from build123d import *

# Parameters (mm, degrees)
SKETCH1_W               = 31.224798093
SKETCH1_H               = 19.847341298
BOSS_EXTRUDE1_DEPTH     = 3.302
SKETCH2_R               = 1.2065
CUT_EXTRUDE1_DEPTH      = 19.847341298
SKETCH3_W               = 6.232143457
SKETCH3_H               = 2.69875
CUT_EXTRUDE2_DEPTH      = 19.847341298
CUT_EXTRUDE4_DEPTH      = 19.847341298
SKETCH6_W               = 7.202949523
SKETCH6_H               = 3.302
CUT_EXTRUDE5_DEPTH      = 19.847341298
SKETCH7_R               = 1.27
CUT_EXTRUDE6_DEPTH      = 0.60325
MIRROR4_COPY_1_SKETCH_R = 1.27
MIRROR4_COPY_1_DEPTH    = 0.60325


with BuildPart() as part:
    # Sketch1 → Boss-Extrude1 (new body)
    with BuildSketch(Plane.XY):
        with Locations((-25.734325238, 15.946701424)):
            Rectangle(SKETCH1_W, SKETCH1_H)
    extrude(amount=BOSS_EXTRUDE1_DEPTH)

    # Sketch2 → Cut-Extrude1 (cut)
    with BuildSketch(Plane.XZ.offset(-6.023030775)):
        with Locations((-25.734325238, 0)):
            Circle(SKETCH2_R)
    extrude(amount=-CUT_EXTRUDE1_DEPTH, mode=Mode.SUBTRACT)

    # Sketch3 → Cut-Extrude2 (cut)
    with BuildSketch(Plane.XZ.offset(-6.023030775)):
        with Locations((-31.390396967, 1.952625)):
            Rectangle(SKETCH3_W, SKETCH3_H)
    cut_extrude2 = extrude(amount=-CUT_EXTRUDE2_DEPTH, mode=Mode.SUBTRACT)

    # Mirror1: Cut-Extrude2 across plane
    add(cut_extrude2.mirror(Plane.ZY.offset(25.734325238)), mode=Mode.SUBTRACT)

    # Sketch5 → Cut-Extrude4 (cut)
    with BuildSketch(Plane.XZ.offset(-6.023030775)):
        with BuildLine():
            Line((-28.274325238, 0.60325), (-28.274325238, 3.302))
            Line((-28.274325238, 3.302), (-23.194325238, 3.302))
            Line((-23.194325238, 3.302), (-23.194325238, 0.60325))
            ThreePointArc((-23.194325238, 0.60325), (-25.734325238, 3.14325), (-28.274325238, 0.60325))
        make_face()
    extrude(amount=-CUT_EXTRUDE4_DEPTH, mode=Mode.SUBTRACT)

    # Sketch6 → Cut-Extrude5 (cut)
    with BuildSketch(Plane.XZ.offset(-6.023030775)):
        with Locations((-37.745249523, 1.651)):
            Rectangle(SKETCH6_W, SKETCH6_H)
    cut_extrude5 = extrude(amount=-CUT_EXTRUDE5_DEPTH, mode=Mode.SUBTRACT)

    # Mirror2: Cut-Extrude5 across plane
    add(cut_extrude5.mirror(Plane.ZY.offset(25.734325238)), mode=Mode.SUBTRACT)

    # Sketch7 → Cut-Extrude6 (cut)
    with BuildSketch(Plane.XY.offset(0.60325)):
        with Locations((-30.814325238, 11.103030775)):
            Circle(SKETCH7_R)
    cut_extrude6 = extrude(amount=-CUT_EXTRUDE6_DEPTH, mode=Mode.SUBTRACT)

    # Mirror3: Cut-Extrude6 across plane
    add(cut_extrude6.mirror(Plane(origin=(0, 15.946701424, 0), x_dir=(0, 0, 1), z_dir=(0, -1, 0))), mode=Mode.SUBTRACT)

    # Mirror4: Cut-Extrude6 across plane
    add(cut_extrude6.mirror(Plane.ZY.offset(25.734325238)), mode=Mode.SUBTRACT)

    # Mirror4 copy 1 sketch → Mirror4 copy 1 (cut)
    with BuildSketch(Plane(origin=(-51.468650475, 31.893402848, 0.60325), x_dir=(-1, 0, 0), z_dir=(0, 0, 1))):
        with Locations((-30.814325238, 11.103030775)):
            Circle(MIRROR4_COPY_1_SKETCH_R)
    extrude(amount=-MIRROR4_COPY_1_DEPTH, mode=Mode.SUBTRACT)


solid = part.part
Design review of the part built by this model. Coordinates are the model's own, in mm. A direction names the side the tool comes from. Round coordinates to 2 decimals unless told otherwise and drop trailing zeros. Write each loop counter-clockwise with the first axis right and the second up, starting at its lowest first coordinate (ties: lowest second). Pieces come first, ordered by that corner, then holes. Notation, with made-up numbers: (-13, 0.5) - (33, 0.5) arc R17 cw to (33, 21.5) - close; hole circle Ø2 at (10.5, -15). An arc over 180 degrees is marked (long way). Use a Markdown table: item, result. Add a question column.
1. Mouldability with a two-part tool opening along Y and no side actions: class faces 1 (the face through (-26, 6.023, 2)), 2 (the face through (-31, 16, 0)), 3 (the face through (-31.09, 9.863, 0.306)) as +Y half, -Y half, draft (parallel to the pull), parting line (faces both ways), or undercut.
2. Clearance check with flat-ended pins moving along their axes: pin 1 (4 mm diameter, centred on x = -20.65, y = 20.79, fed in from +Z); pin 2 (1 mm diameter, centred on y = 17, z = 1.5, fed in from -X); pin 3 (1.5 mm diameter, centred on x = -25.5, y = 16.5, fed in from -Z). State where each tip first meets the part, or that it passes through.
3. We need section B-B (y = 24). State the section outline as (x, z) points, then the cut area to 3 significant figures.
4. For faces 4 (the face through (-31, 16, 0.603)), 5 (the face through (-20.49, 19.53, 0.31)), 6 (the face through (-20, 16, 0.603)), list the 3-axis set-ups (+Z, -Z, +X, -X, +Y, -Y) from which the entire face can be reached by the end or side of a thin tool; tool diameter is ignored.
5. We need section C-C (x = -21). State the section outline as (y, z) points, then the cut area to 3 significant figures.
6. We need section A-A (z = 0.3). State the section outline as (x, y) points, then the cut area to 3 significant figures.
7. Wall thickness on probe 1 along Y at (x, z) = (-19.5, 0.35); probe 2 along Y at (x, z) = (-30.75, 0.3); probe 3 along Z at (x, y) = (-32.25, 21.5): over which ranges is each line inside the solid? List them lowest first.
8. We need section D-D (y = 21.5). State the section outline as (x, z) points, then the cut area to 3 significant figures.
Output:
| question | item | result |
|---|---|---|
| 1 | face 1 | -Y half |
| 1 | face 2 | draft |
| 1 | face 3 | undercut |
| 2 | pin 1 | stops at z = 0.6 |
| 2 | pin 2 | stops at x = -28.24 |
| 2 | pin 3 | stops at z = 0.7 |
| 3 | outline | (-34.14, 0) - (-26.94, 0) arc R1.21 cw to (-24.53, 0) - (-17.32, 0) - (-17.32, 0.6) - (-23.19, 0.6) arc R2.54 ccw to (-28.27, 0.6) - (-34.14, 0.6) - close |
| 3 | area | 18.0 mm2 |
| 4 | face 4 | +Z, -X, +Y, -Y |
| 4 | face 5 | +Z, -Z |
| 4 | face 6 | +Z, +X, +Y, -Y |
| 5 | outline | (6.02, 0) - (9.88, 0) - (9.88, 0.6) - (6.02, 0.6) - close; (12.33, 0) - (19.57, 0) - (19.57, 0.6) - (12.33, 0.6) - close; (22.01, 0) - (25.87, 0) - (25.87, 0.6) - (22.01, 0.6) - close |
| 5 | area | 9.02 mm2 |
| 6 | outline | (-34.14, 6.02) - (-26.9, 6.02) - (-26.9, 25.87) - (-34.14, 25.87) - close; (-24.57, 6.02) - (-17.32, 6.02) - (-17.32, 25.87) - (-24.57, 25.87) - close; hole circle Ø2.54 at (-30.81, 11.1); hole circle Ø2.54 at (-30.81, 20.79); hole circle Ø2.54 at (-20.65, 11.1); hole circle Ø2.54 at (-20.65, 20.79) |
| 6 | area | 267 mm2 |
| 7 | probe 1 | y = 6.02 to 10.57, 11.63 to 20.26, 21.32 to 25.87 |
| 7 | probe 2 | y = 6.02 to 9.83, 12.37 to 19.52, 22.06 to 25.87 |
| 7 | probe 3 | z = 0 to 0.6 |
| 8 | outline | (-34.14, 0) - (-31.87, 0) - (-31.87, 0.6) - (-34.14, 0.6) - close; (-29.76, 0) - (-26.94, 0) arc R1.21 cw to (-24.53, 0) - (-21.71, 0) - (-21.71, 0.6) - (-23.19, 0.6) arc R2.54 ccw to (-28.27, 0.6) - (-29.76, 0.6) - close; (-19.6, 0) - (-17.32, 0) - (-17.32, 0.6) - (-19.6, 0.6) - close |
| 8 | area | 15.5 mm2 |
